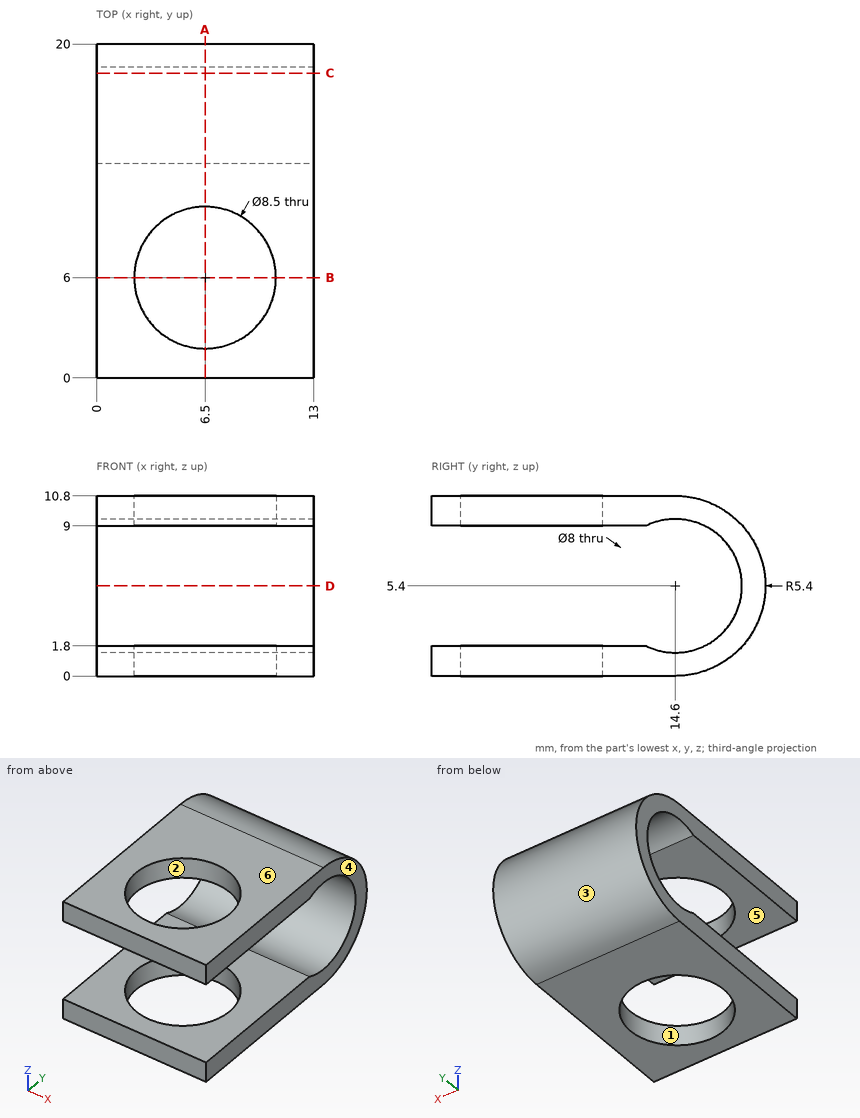
The drawing under review shows one solid part. Ordinate dimensions are in mm from its lowest x, y, z. A direction names the side the tool comes from. Coordinates: 2 decimals unless noted, no trailing zeros. Order: outer loops, then holes, each group sorted by start corner. A loop starts at its lowest first (then second) coordinate and runs counter-clockwise, first axis right, second up. Notation, with made-up numbers: (2, 65) -> (39, 65) arc R22 ccw to (39, 101) -> close; hole circle Ø3 at (-31, 56). An arc over 180 degrees is marked (long way). Answer in a Markdown table with one row per item.
(1) Insertion check: pin 1 (1 mm diameter, centred on y = 10.5, z = 2.5, fed in from -X). The pin has a flat end and moves straight along its axis. Give the tip position at first contact, or say it passes through.
Answers:
| item | result |
|---|---|
| pin 1 | through |
(2) Consider section B-B (y = 6). Write out the cut boundary in (x, z).
Answers:
| item | result |
|---|---|
| outline | (0, 0) -> (2.25, 0) -> (2.25, 1.8) -> (0, 1.8) -> close; (0, 9) -> (2.25, 9) -> (2.25, 10.8) -> (0, 10.8) -> close; (10.75, 0) -> (13, 0) -> (13, 1.8) -> (10.75, 1.8) -> close; (10.75, 9) -> (13, 9) -> (13, 10.8) -> (10.75, 10.8) -> close |
(3) Consider section C-C (y = 18.25). Write out the cut boundary in (x, z), plus the area to 3 significant figures.
Answers:
| item | result |
|---|---|
| outline | (0, 1.42) -> (13, 1.42) -> (13, 3.76) -> (0, 3.76) -> close; (0, 7.04) -> (13, 7.04) -> (13, 9.38) -> (0, 9.38) -> close |
| area | 60.9 mm² |
(4) Consider section D-D (z = 5.4). Write out the cut boundary in (x, y), plus the area to 3 significant figures.
Answers:
| item | result |
|---|---|
| outline | (0, 18.6) -> (13, 18.6) -> (13, 20) -> (0, 20) -> close |
| area | 18.2 mm² |
(5) The part is to be moulded in two halves that separate along Y. For the marked faces 1, 2, 3 and 4, say which applies: +Y half, -Y half, draft (parallel to the pull), parting line (faces both ways), or undercut.
Answers:
| item | result |
|---|---|
| face 1 | undercut |
| face 2 | undercut |
| face 3 | +Y half |
| face 4 | draft |
(6) Machinability: for the marked faces 5 and 6, which of the approach directions +Z, -Z, +X, -X, +Y, -Y give a long, thin tool a straight path to every point of the face, cutting with its end or side? Answer none if there is none.
Answers:
| item | result |
|---|---|
| face 5 | +X, -X, -Y |
| face 6 | +Z, +X, -X, +Y, -Y |
(7) Wall thickness on line 1 along Z through (x, y) = (10, 14.6); line 2 along Z through (x, y) = (8.5, 11.75); line 3 along Y through (x, z) = (5, 1): over which ranges is each line inside the solid? List them lowest first.
Answers:
| item | result |
|---|---|
| line 1 | 0 to 1.4, 9.4 to 10.8 |
| line 2 | 0 to 1.8, 9 to 10.8 |
| line 3 | 0 to 2.02, 9.98 to 17.73 |
(8) Consider section A-A (x = 6.5). Write out the cut boundary in (y, z).
Answers:
| item | result |
|---|---|
| outline | (0, 0) -> (1.75, 0) -> (1.75, 1.8) -> (0, 1.8) -> close; (0, 9) -> (1.75, 9) -> (1.75, 10.8) -> (0, 10.8) -> close; (10.25, 0) -> (14.6, 0) arc R5.4 ccw to (14.6, 10.8) -> (10.25, 10.8) -> (10.25, 9) -> (12.86, 9) arc R4 cw (long way) to (12.86, 1.8) -> (10.25, 1.8) -> close |
